Read the model definition and answer for the solid it produces. Units are mm, in the model's axes. A direction names the side the tool comes from. Give positions to 0.01 mm unless a question says otherwise; leave off trailing zeros. Order: outer loops, then holes, each group sorted by start corner. A loop starts at its lowest first (then second) coordinate and runs counter-clockwise, first axis right, second up. Notation, with made-up numbers: (81.5, 62) - (123.5, 62) arc R21 cw to (123.5, 76) - close; hole circle Ø3 at (15.25, 83.25). An arc over 180 degrees is marked (long way). Return JSON: item names as keys, results as strings.
```python
from build123d import *

# Parameters (mm, degrees)
F0_W     = 76.2
F0_H     = 76.2
F1_DEPTH = 19.05
F2_R     = 25.4
F3_DEPTH = 76.2
F4_W     = 76.2
F4_H     = 76.2
F4_R     = 25.4
F5_DEPTH = 19.05
F6_R     = 19.05
F7_DEPTH = 114.3
F9_DEPTH = 127


with BuildPart() as f1:
    # F0 (on Front) → F1 (new body)
    with BuildSketch(Plane.XZ):
        Rectangle(F0_W, F0_H)
    extrude(amount=F1_DEPTH)

    # F2 (on face) → F3 (join)
    with BuildSketch(Plane.XZ.offset(19.05)):
        Circle(F2_R)
    extrude(amount=F3_DEPTH)

    # F4 (on face) → F5 (join)
    with BuildSketch(Plane.XZ.offset(95.25)):
        Rectangle(F4_W, F4_H)
        Circle(F4_R, mode=Mode.SUBTRACT)
        Circle(F4_R)
    extrude(amount=F5_DEPTH)

    # F6 (on face) → F7 (cut)
    with BuildSketch(Plane.XZ.offset(114.3)):
        Circle(F6_R)
    extrude(amount=-F7_DEPTH, mode=Mode.SUBTRACT)

    # F8 (on face) → F9 (cut)
    with BuildSketch(Plane.XZ.offset(114.3)):
        with BuildLine():
            ThreePointArc((-22.225, 28.575), (-24.0848719395, 33.0651280605), (-28.575, 34.925))
            ThreePointArc((-28.575, 34.925), (-33.0651280605, 24.0848719395), (-22.225, 28.575))
        make_face()
        with BuildLine():
            ThreePointArc((-22.225, -28.575), (-33.0651280605, -24.0848719395), (-28.575, -34.925))
            ThreePointArc((-28.575, -34.925), (-24.0848719395, -33.0651280605), (-22.225, -28.575))
        make_face()
        with BuildLine():
            ThreePointArc((34.925, -28.575), (24.0848719395, -24.0848719395), (28.575, -34.925))
            ThreePointArc((28.575, -34.925), (33.0651280605, -33.0651280605), (34.925, -28.575))
        make_face()
        with BuildLine():
            ThreePointArc((34.925, 28.575), (33.0651280605, 33.0651280605), (28.575, 34.925))
            ThreePointArc((28.575, 34.925), (24.0848719395, 24.0848719395), (34.925, 28.575))
        make_face()
    extrude(amount=-F9_DEPTH, mode=Mode.SUBTRACT)


solid = f1.part
```
Q1. A cutting plane is placed at A-A (z = 0). Write down the section's boundary in (x, y), and give its area (3 significant figures).
Values:
{"outline": "(-38.1, -114.3) - (-19.05, -114.3) - (-19.05, 0) - (-38.1, 0) - (-38.1, -19.05) - (-25.4, -19.05) - (-25.4, -95.25) - (-38.1, -95.25) - close; (19.05, -114.3) - (38.1, -114.3) - (38.1, -95.25) - (25.4, -95.25) - (25.4, -19.05) - (38.1, -19.05) - (38.1, 0) - (19.05, 0) - close", "area": "2,420 mm²"}
Q2. For faces 4 (the flat face through (-38.1, -9, -1)), 5 (the flat face through (-1, -95.25, 26)), determine the directions among +Z, -Z, +X, -X, +Y, -Y from which every point of the face is accessible in a straight line to the end or side of a thin tool.
Values:
{"face 4": "+Z, -Z, -X, +Y, -Y", "face 5": "none"}
Q3. A cutting plane is placed at B-B (x = 0). Write down the section's boundary in (y, z).
Values:
{"outline": "(-114.3, -38.1) - (-95.25, -38.1) - (-95.25, -25.4) - (-19.05, -25.4) - (-19.05, -38.1) - (0, -38.1) - (0, -19.05) - (-114.3, -19.05) - close; (-114.3, 19.05) - (0, 19.05) - (0, 38.1) - (-19.05, 38.1) - (-19.05, 25.4) - (-95.25, 25.4) - (-95.25, 38.1) - (-114.3, 38.1) - close"}
Q4. A cutting plane is placed at D-D (y = -50.5). Write down the section's boundary in (x, z), and give its area (3 significant figures).
Values:
{"outline": "circle Ø50.8 at (0, 0); hole circle Ø38.1 at (0, 0)", "area": "887 mm²"}
Q5. A cutting plane is placed at C-C (z = -32). Write down the section's boundary in (x, y), and give its area (3 significant figures).
Values:
{"outline": "(-38.1, -114.3) - (-33.92, -114.3) - (-33.92, -95.25) - (-38.1, -95.25) - close; (-38.1, -19.05) - (-33.92, -19.05) - (-33.92, 0) - (-38.1, 0) - close; (-23.23, -114.3) - (23.23, -114.3) - (23.23, -95.25) - (-23.23, -95.25) - close; (-23.23, -19.05) - (23.23, -19.05) - (23.23, 0) - (-23.23, 0) - close; (33.92, -114.3) - (38.1, -114.3) - (38.1, -95.25) - (33.92, -95.25) - close; (33.92, -19.05) - (38.1, -19.05) - (38.1, 0) - (33.92, 0) - close", "area": "2,090 mm²"}
Q6. Consider L1, parallel to Y at x = 32.5, z = 20; L2, parallel to Z at x = -30, y = -9; L3, parallel to Z at x = 0.5, y = -81. Determine where each line is inside the solid, lowest interval first.
Values:
{"L1": "y = -114.3 to -95.25, -19.05 to 0", "L2": "z = -38.1 to -34.76, -22.39 to 22.39, 34.76 to 38.1", "L3": "z = -25.4 to -19.04, 19.04 to 25.4"}
Q7. Determine the mould class of faces 1 (the flat face through (-1, -19.05, 26)), 2 (the flat face through (-9, 0, 17)), 3 (the cylindrical face through (-15.12, -57.95, -11.59)) for opening direction Y: released by +Y, released by -Y, zero draft, split by the parting line, or undercut.
Values:
{"face 1": "undercut", "face 2": "released by +Y", "face 3": "zero draft"}
Q8. Given pin 1 (5 mm diameter, centred on x = -14.5, y = -59.5, fed in from -Z); pin 2 (1.5 mm diameter, centred on x = 12, y = -44.5, fed in from -Z), each flat-ended and moving along its own axis, determine where each tip first touches the part or whether it passes through.
Values:
{"pin 1": "stops at z = -22.39", "pin 2": "stops at z = -22.77"}
